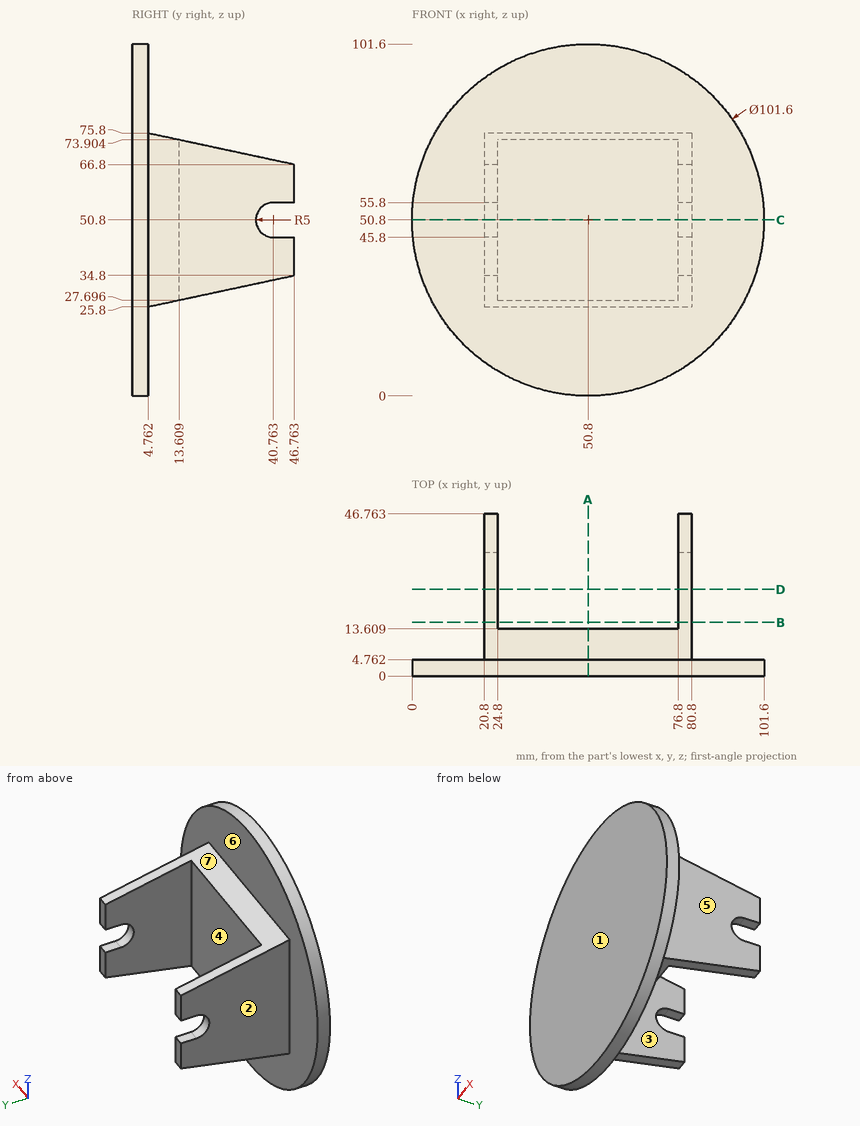
The drawing under review shows one solid part. Ordinate dimensions are in mm from its lowest x, y, z. A direction names the side the tool comes from. Round coordinates to 2 decimals unless told otherwise and drop trailing zeros. Loops run counter-clockwise (first coordinate to the right, second up) from the corner with the lowest first, then second, coordinate; pieces in that order, holes last. Notation, with made-up numbers: M 46,46 L 103,46 A26 cw 103,66 Z; hole C -15.75,33 d5. An arc over 180 degrees is marked long. Answer as CSV lines item,"result". Start each with the question number.
Item 1: For the marked faces 4, 5, 6 and 7, list the 3-axis set-ups (+Z, -Z, +X, -X, +Y, -Y) from which the entire face can be reached by the end or side of a thin tool; tool diameter is ignored.
Item 2: Insertion check: P1, Ø16.5, axis at y = 31, z = 41.5, coming from the -X side; P2, Ø10, axis at x = 73.5, y = 12, coming from the +Z side; P3, Ø1.2, axis at x = 22.5, y = 43, coming from the -Z side (1 decimal). Each pin has a flat end and moves straight along its axis. Give the tip position at first contact, or say it passes through.
Item 3: Consider section B-B (y = 15.5). Write out the cut boundary in (x, z), then the cut area to 3 significant figures.
Item 4: Consider section A-A (x = 50.8). Write out the cut boundary in (y, z) (1 decimal).
Item 5: Consider section C-C (z = 50.8). Write out the cut boundary in (x, y).
Item 6: Wall thickness on line 1 (X direction, y = 28.5, z = 33); line 2 (Y direction, x = 27, z = 44.5); line 3 (Y direction, x = 93.5, z = 69): over which ranges is each line inside the solid? List them lowest first. Write a range as [from, to].
Item 7: Mouldability with a two-part tool opening along X and no side actions: class the marked faces 1, 2 and 3 as released by +X, released by -X, zero draft, split by the parting line, or undercut.
Item 8: Consider section D-D (y = 25). Write out the cut boundary in (x, z).
Answer:
1,face 4,"+Z, -Z, +Y"
1,face 5,"+Z, -Z, +X, +Y"
1,face 6,"+Y"
1,face 7,"+Z, +X, -X, +Y"
2,P1,"stops at x = 20.8"
2,P2,"stops at z = 75.32"
2,P3,"stops at z = 33.9"
3,outline,"M 20.8,28.1 L 24.8,28.1 L 24.8,73.5 L 20.8,73.5 Z; M 76.8,28.1 L 80.8,28.1 L 80.8,73.5 L 76.8,73.5 Z"
3,area,"363 mm^2"
4,outline,"M 0,0 L 4.8,0 L 4.8,25.8 L 13.6,27.7 L 13.6,73.9 L 4.8,75.8 L 4.8,101.6 L 0,101.6 Z"
5,outline,"M 0,0 L 101.6,0 L 101.6,4.76 L 80.8,4.76 L 80.8,35.76 L 76.8,35.76 L 76.8,13.61 L 24.8,13.61 L 24.8,35.76 L 20.8,35.76 L 20.8,4.76 L 0,4.76 Z"
6,line 1,"x = [20.8, 24.8], [76.8, 80.8]"
6,line 2,"y = [0, 13.61]"
6,line 3,"y = [0, 4.76]"
7,face 1,"zero draft"
7,face 2,"released by -X"
7,face 3,"undercut"
8,outline,"M 20.8,30.14 L 24.8,30.14 L 24.8,71.46 L 20.8,71.46 Z; M 76.8,30.14 L 80.8,30.14 L 80.8,71.46 L 76.8,71.46 Z"
